from build123d import *

# Parameters (mm, degrees)
SKETCH1_W                          = 28
SKETCH1_H                          = 20
BOSS_EXTRUDE1_DEPTH                = 3
F_3_0_3_DIAMETER_HOLE7_D           = 3
F_3_0_3_DIAMETER_HOLE7_DEPTH       = 3
F_3_0_3_DIAMETER_HOLE7_CSINK_D     = 3.05
F_3_0_3_DIAMETER_HOLE7_CSINK_ANGLE = 90
F_3_0_3_DIAMETER_HOLE7_TIP         = 0.901290929


with BuildPart() as part:
    # Sketch1 → Boss-Extrude1 (new body)
    with BuildSketch(Plane(origin=(0, 0, 0), x_dir=(1, 0, 0), z_dir=(0, 1, 0))):
        Rectangle(SKETCH1_W, SKETCH1_H)
    extrude(amount=-BOSS_EXTRUDE1_DEPTH)

    # Ø3.0 (3) Diameter Hole7
    with Locations(Plane(origin=(0, 0, 0), x_dir=(1, 0, 0), z_dir=(0, 1, 0))):
        with Locations((-10.5, 7.545553469), (10.5, 7.545553469), (10.5, -6.860504487), (-10.5, -6.860504487)):
            CounterSinkHole(F_3_0_3_DIAMETER_HOLE7_D / 2, F_3_0_3_DIAMETER_HOLE7_CSINK_D / 2, depth=F_3_0_3_DIAMETER_HOLE7_DEPTH, counter_sink_angle=F_3_0_3_DIAMETER_HOLE7_CSINK_ANGLE)
            with Locations((0, 0, -(F_3_0_3_DIAMETER_HOLE7_DEPTH + F_3_0_3_DIAMETER_HOLE7_TIP / 2))):  # 118° drill point
                Cone(0, F_3_0_3_DIAMETER_HOLE7_D / 2, F_3_0_3_DIAMETER_HOLE7_TIP, mode=Mode.SUBTRACT)


solid = part.part
Source: CAD feature listing. Evaluate the final solid. Frame: model axes, mm. Give positions to 0.01 mm unless a question says otherwise; leave off trailing zeros. Write each loop counter-clockwise with the first axis right and the second up, starting at its lowest first coordinate (ties: lowest second). Pieces come first, ordered by that corner, then holes. Notation, with made-up numbers: M -14.75,32.25 L -1.75,32.25 A19 ccw -1.75,51.25 Z; hole C 76,-22 d4. An arc over 180 degrees is marked long. Return JSON: item names as keys, results as strings. Group by question number.
1) Cut plane A-A, the plane x = 10.5. Give the number of separate pieces and of enclosed holes in the cut face, plus the area to 3 significant figures.
2) Pin query (flat end, axial travel): P1, Ø2.5, axis at x = -10.5, z = -7.55, coming from the -Y side. Return the tip coordinate at first contact, or that it passes through.
3) Pull-direction query (Z, two-part tool) for faces 1 (the face through (0, -1, 10)), 2 (the face through (10.825, -1.533, 8.325)), 3 (the face through (-9.394, -1.533, -8.559)), 4 (the face through (14, -1, 0)); classes: pulls with the +Z half, pulls with the -Z half, needs draft (parallel to the pull), parting line crosses it, or undercut.
4) Cut plane B-B, the plane y = -0.8. Output: boundary loops of the cut face in (x, z), plus the area to 3 significant figures.
5) Material intervals for line 1 along Z through (x, y) = (-10.5, -1.1); line 2 along X through (y, z) = (-2.6, 7); line 3 along Z through (x, y) = (-11.5, -1.7), sorted ascending. Write a range as [from, to].
Recorded:
{
 "1": {"separate pieces": "3", "enclosed holes": "0", "area": "42.0 mm²"},
 "2": {"P1": "passes through"},
 "3": {"face 1": "pulls with the +Z half", "face 2": "undercut", "face 3": "undercut", "face 4": "needs draft"},
 "4": {"outline": "M -14,-10 L 14,-10 L 14,10 L -14,10 Z; hole C -10.5,-7.55 d3; hole C -10.5,6.86 d3; hole C 10.5,-7.55 d3; hole C 10.5,6.86 d3", "area": "532 mm²"},
 "5": {"line 1": "z = [-10, -9.05], [-6.05, 5.36], [8.36, 10]", "line 2": "x = [-14, -11.99], [-9.01, 9.01], [11.99, 14]", "line 3": "z = [-10, -8.66], [-6.43, 5.74], [7.98, 10]"}
}
